```python
from build123d import *

# Parameters (mm, degrees)
SKETCH1_W           = 71
SKETCH1_H           = 12
BOSS_EXTRUDE1_DEPTH = 2
SKETCH2_R           = 2.5
SKETCH2_R_2         = 1.625
BOSS_EXTRUDE2_DEPTH = 2


with BuildPart() as part:
    # Sketch1 → Boss-Extrude1 (new body)
    with BuildSketch(Plane.XY):
        with Locations((35.5, 6)):
            Rectangle(SKETCH1_W, SKETCH1_H)
    extrude(amount=BOSS_EXTRUDE1_DEPTH)

    # Sketch2 → Boss-Extrude2 (add)
    # profile 1 of 2: a face of its own
    with BuildSketch(Plane.XY.offset(2)):
        with Locations(Location((19, 6, 0), (0, 0, 180))):
            Circle(SKETCH2_R)
        with Locations((19, 6)):
            Circle(SKETCH2_R_2, mode=Mode.SUBTRACT)
    # profile 2 of 2: a face of its own
    with BuildSketch(Plane.XY.offset(2)):
        with Locations(Location((49, 6, 0), (0, 0, 180))):
            Circle(SKETCH2_R)
        with Locations((49, 6)):
            Circle(SKETCH2_R_2, mode=Mode.SUBTRACT)
    extrude(amount=BOSS_EXTRUDE2_DEPTH)


solid = part.part
```
Here's how the part is built. I have some questions about the finished solid (model axes, mm). A direction names the side the tool comes from. Coordinates: 2 decimals unless noted, no trailing zeros. Order: outer loops, then holes, each group sorted by start corner. A loop starts at its lowest first (then second) coordinate and runs counter-clockwise, first axis right, second up.
1) Which directions (+Z, -Z, +X, -X, +Y, -Y) give clear straight access to the entire face, cutting with the end or side of a thin tool? Please do faces 1 (the face through (20.55, 6.49, 2.99)), 2 (the face through (35, 6, 0)).
2) Imagine slicing it at C-C on y = 7. List the corners of the cut face in (x, z) for me.
3) We'd pull the mould along X, two halves only. Please class faces 3 (the face through (71, 6, 1)), 4 (the face through (0, 6, 1)), 5 (the face through (47, 6, 4)), 6 (the face through (21.5, 5.9, 3)): +X half, -X half, draft (parallel to the pull), parting line (faces both ways), or undercut.
4) Imagine slicing it at D-D on x = 7. List the corners of the cut face in (y, z) for me, and give its area (3 significant figures).
5) I need wall thicknesses on line 1 (Y direction, x = 19, z = 2.65) (3 decimals); line 2 (X direction, y = 4.75, z = 3); line 3 (X direction, y = 6.75, z = 2.15). Which ranges of each line are inside material? Lowest first, please.
6) Imagine slicing it at A-A on z = 3.3. List the corners of the cut face in (x, y) for me (3 decimals), and give its area (3 significant figures).
7) Imagine slicing it at B-B on x = 19. List the corners of the cut face in (y, z) for me (3 decimals), and give its area (3 significant figures).
8) Will these pins go through, and if not, where does the flat tip stop? pin 1 (1.6 mm diameter, centred on x = 49.5, y = 6.5, fed in from +Z); pin 2 (6 mm diameter, centred on x = 22.5, y = 7, fed in from +Z).
Response values:
1. face 1: +Z
1. face 2: -Z, +X, -X, +Y, -Y
2. outline: (0, 0) - (71, 0) - (71, 2) - (51.29, 2) - (51.29, 4) - (50.28, 4) - (50.28, 2) - (47.72, 2) - (47.72, 4) - (46.71, 4) - (46.71, 2) - (21.29, 2) - (21.29, 4) - (20.28, 4) - (20.28, 2) - (17.72, 2) - (17.72, 4) - (16.71, 4) - (16.71, 2) - (0, 2) - close
3. face 3: +X half
3. face 4: -X half
3. face 5: draft
3. face 6: undercut
4. outline: (0, 0) - (12, 0) - (12, 2) - (0, 2) - close
4. area: 24.0 mm2
5. line 1: y = 3.5 to 4.375, 7.625 to 8.5
5. line 2: x = 16.83 to 17.96, 20.04 to 21.17, 46.83 to 47.96, 50.04 to 51.17
5. line 3: x = 16.62 to 17.56, 20.44 to 21.38, 46.62 to 47.56, 50.44 to 51.38
6. outline: circle Ø5 at (19, 6); circle Ø5 at (49, 6); hole circle Ø3.25 at (19, 6); hole circle Ø3.25 at (49, 6)
6. area: 22.7 mm2
7. outline: (0, 0) - (12, 0) - (12, 2) - (8.5, 2) - (8.5, 4) - (7.625, 4) - (7.625, 2) - (4.375, 2) - (4.375, 4) - (3.5, 4) - (3.5, 2) - (0, 2) - close
7. area: 27.5 mm2
8. pin 1: stops at z = 2
8. pin 2: stops at z = 4
